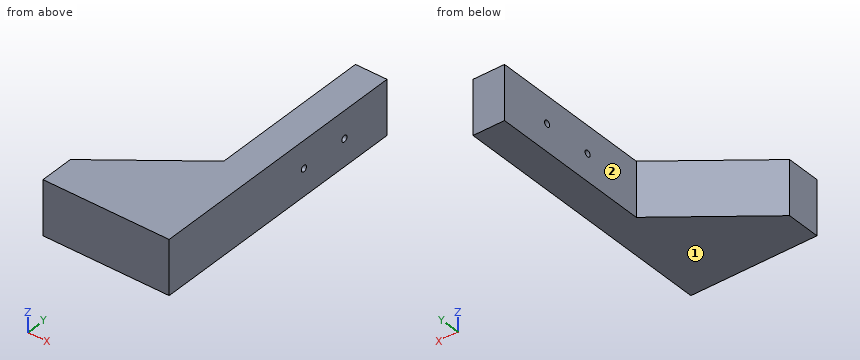
```python
from build123d import *

# Parameters (mm, degrees)
BOSS_EXTRUDE1_DEPTH = 43
SKETCH2_R           = 2.5
CUT_EXTRUDE1_DEPTH  = 25


with BuildPart() as part:
    # Sketch1 → Boss-Extrude1 (new body)
    with BuildSketch(Plane.XY):
        Polygon((0, 0), (0, 130), (25, 130), (25, -85), (-75, -85), (-75, -58), align=None)
    extrude(amount=BOSS_EXTRUDE1_DEPTH)

    # Sketch2 → Cut-Extrude1 (cut)
    with BuildSketch(Plane.ZY):
        with Locations((21.5, 88)):
            Circle(SKETCH2_R)
        with Locations((21.5, 48)):
            Circle(SKETCH2_R)
    extrude(amount=-CUT_EXTRUDE1_DEPTH, mode=Mode.SUBTRACT)


solid = part.part
```
Geometry: final body of the model. Coordinates: model frame, mm. Face numbers are marked on the shaded views. A direction names the side the tool comes from. Round coordinates to 2 decimals unless told otherwise and drop trailing zeros. Order: outer loops, then holes, each group sorted by start corner. A loop starts at its lowest first (then second) coordinate and runs counter-clockwise, first axis right, second up. Notation, with made-up numbers: (87, 54) -> (95, 54) arc R19 cw to (95, 66) -> close; hole circle Ø6 at (61, -9.5). An arc over 180 degrees is marked (long way). Write each question's results on one line, items separated by ' | '.
Q1. Section query D-D (y = -49.5). Output: boundary loops of the cut face in (x, z), and give its area (3 significant figures).
Response values:
outline: (-64.01, 0) -> (25, 0) -> (25, 43) -> (-64.01, 43) -> close | area: 3,830 mm²
Q2. Ray query, line 1 along Y through (x, z) = (17.5, 21.5); line 2 along Y through (x, z) = (8.5, 22); line 3 along X through (y, z) = (88, 15.5). Return the intervals inside material, ascending.
Response values:
line 1: -85 to 45.5, 50.5 to 85.5, 90.5 to 130 | line 2: -85 to 45.55, 50.45 to 85.55, 90.45 to 130 | line 3: 0 to 25
Q3. Section query C-C (x = -3). Output: boundary loops of the cut face in (y, z), and give its area (3 significant figures).
Response values:
outline: (-85, 0) -> (-2.32, 0) -> (-2.32, 43) -> (-85, 43) -> close | area: 3,560 mm²
Q4. Pin query (flat end, axial travel): pin 1 Ø6.5 at (y, z) = (88, 21.5) entering from -X; pin 2 Ø6 at (y, z) = (-54, 38.5) entering from -X; pin 3 Ø4 at (y, z) = (48, 21.5) entering from -X; pin 4 Ø8 at (x, y) = (-2.5, 76.5) entering from -Z. Return the tip coordinate at first contact, or that it passes through.
Response values:
pin 1: x = 0 | pin 2: x = -73.71 | pin 3: through | pin 4: z = 0
Q5. Section query A-A (z = 21.5). Output: boundary loops of the cut face in (x, y).
Response values:
outline: (-75, -85) -> (25, -85) -> (25, 45.5) -> (0, 45.5) -> (0, 0) -> (-75, -58) -> close; (0, 50.5) -> (25, 50.5) -> (25, 85.5) -> (0, 85.5) -> close; (0, 90.5) -> (25, 90.5) -> (25, 130) -> (0, 130) -> close
Q6. Access query for the marked faces 1 and 2. Directions: +Z, -Z, +X, -X, +Y, -Y. A direction counts if a zero-diameter tool reaches every point of the face in a straight line with its end or side. Return the directions, or none.
Response values:
face 1: -Z, +X, -X, +Y, -Y | face 2: +Z, -Z, -X, +Y
Q7. Section query B-B (y = 48). Output: boundary loops of the cut face in (x, z), and give its area (3 significant figures).
Response values:
outline: (0, 0) -> (25, 0) -> (25, 19) -> (0, 19) -> close; (0, 24) -> (25, 24) -> (25, 43) -> (0, 43) -> close | area: 950 mm²
